from build123d import *

# Parameters (mm, degrees)
BOSS_EXTRUDE1_DEPTH                             = 38.1
BOSS_EXTRUDE2_START                             = -3.175
BOSS_EXTRUDE2_DEPTH                             = 3.175
CBORE_FOR_2_PAN_HEAD_MACHINE_SCREW1_D           = 2.7051
CBORE_FOR_2_PAN_HEAD_MACHINE_SCREW1_DEPTH       = 2.667
CBORE_FOR_2_PAN_HEAD_MACHINE_SCREW1_CBORE_D     = 4.7625
CBORE_FOR_2_PAN_HEAD_MACHINE_SCREW1_CBORE_DEPTH = 1.5748
CBORE_START                                     = 26.4287
CBORE_FOR_2_PAN_HEAD_MACHINE_SCREW2_OUT_R       = 2.38125
CBORE_FOR_2_PAN_HEAD_MACHINE_SCREW2_DEPTH       = 1.574800075
CBORE_START_2                                   = 25.300372244
CBORE_FOR_2_PAN_HEAD_MACHINE_SCREW2_2_O_R       = 1.35255
CBORE_FOR_2_PAN_HEAD_MACHINE_SCREW2_2_DEPTH     = 1.128327756
CBORE_START_3                                   = -28.003500101
CBORE_FOR_2_PAN_HEAD_MACHINE_SCREW3_OUT_R       = 2.38125
CBORE_FOR_2_PAN_HEAD_MACHINE_SCREW3_DEPTH       = 1.574800101
CBORE_START_4                                   = -26.4287
CBORE_FOR_2_PAN_HEAD_MACHINE_SCREW3_2_O_R       = 1.35255
CBORE_FOR_2_PAN_HEAD_MACHINE_SCREW3_2_DEPTH     = 1.128327733
CUT_EXTRUDE1_REACH                              = 56.955
SKETCH20_R                                      = 7.27
HOLE1_AT_2_COUNT                                = 2
HOLE1_AT_2_PITCH                                = 19
F_0_CLEARANCE_HOLE1_D                           = 1.8542
CHAMFER1_SIZE                                   = 1.27


# Read off the part's stored shape, not the designer's step: CBORE for #2 Pan Head Machine Screw2, CBORE for #2 Pan Head Machine Screw3
with BuildPart() as part:
    # Sketch1 → Boss-Extrude1 (new body)
    with BuildSketch(Plane.XY):
        with BuildLine():
            Line((15.182514888, 23.53056), (-15.182514888, 23.53056))
            ThreePointArc((-15.182514888, 23.53056), (0, -28.0035), (15.182514888, 23.53056))
        make_face()
        with BuildLine():
            Line((14.375329435, 20.86356), (-14.375329435, 20.86356))
            ThreePointArc((-14.375329435, 20.86356), (0, -25.3365), (14.375329435, 20.86356))
        make_face(mode=Mode.SUBTRACT)
    extrude(amount=BOSS_EXTRUDE1_DEPTH)

    # Sketch10 → Boss-Extrude2 (add)
    with BuildSketch(Plane.XY.offset(38.1).offset(BOSS_EXTRUDE2_START)):
        with BuildLine():
            Line((15.182514888, 23.53056), (-15.182514888, 23.53056))
            ThreePointArc((-15.182514888, 23.53056), (0, -28.0035), (15.182514888, 23.53056))
        make_face()
    extrude(amount=BOSS_EXTRUDE2_DEPTH)

    # CBORE for #2 Pan Head Machine Screw1
    with Locations(Plane(origin=(-7.747359339, 23.53056, 10.2108), x_dir=(0, 0, -1), z_dir=(0, 1, 0))):
        with Locations((1.8613, -7.747359339)):
            CounterBoreHole(CBORE_FOR_2_PAN_HEAD_MACHINE_SCREW1_D / 2, CBORE_FOR_2_PAN_HEAD_MACHINE_SCREW1_CBORE_D / 2, CBORE_FOR_2_PAN_HEAD_MACHINE_SCREW1_CBORE_DEPTH, depth=CBORE_FOR_2_PAN_HEAD_MACHINE_SCREW1_DEPTH)

    # CBORE for #2 Pan Head Machine Screw2 out → CBORE for #2 Pan Head Machine Screw2 (cut)
    with BuildSketch(Plane(origin=(0, 0, 0), x_dir=(0.8660254037844416, 0.4999999999999948, 0), z_dir=(0.4999999999999948, -0.8660254037844417, 0)).offset(CBORE_START)):
        with Locations((0, 10.2108)):
            Circle(CBORE_FOR_2_PAN_HEAD_MACHINE_SCREW2_OUT_R)
    extrude(amount=CBORE_FOR_2_PAN_HEAD_MACHINE_SCREW2_DEPTH, mode=Mode.SUBTRACT)

    # CBORE for _2 Pan Head Machine Screw2 2 o → CBORE for _2 Pan Head Machine Screw2 2 (cut)
    with BuildSketch(Plane(origin=(0, 0, 0), x_dir=(0.8660254037844416, 0.4999999999999948, 0), z_dir=(0.4999999999999948, -0.8660254037844417, 0)).offset(CBORE_START_2)):
        with Locations((0, 10.2108)):
            Circle(CBORE_FOR_2_PAN_HEAD_MACHINE_SCREW2_2_O_R)
    extrude(amount=CBORE_FOR_2_PAN_HEAD_MACHINE_SCREW2_2_DEPTH, mode=Mode.SUBTRACT)

    # CBORE for #2 Pan Head Machine Screw3 out → CBORE for #2 Pan Head Machine Screw3 (cut)
    with BuildSketch(Plane.YZ.offset(CBORE_START_3)):
        with Locations((0, 10.2108)):
            Circle(CBORE_FOR_2_PAN_HEAD_MACHINE_SCREW3_OUT_R)
    extrude(amount=CBORE_FOR_2_PAN_HEAD_MACHINE_SCREW3_DEPTH, mode=Mode.SUBTRACT)

    # CBORE for _2 Pan Head Machine Screw3 2 o → CBORE for _2 Pan Head Machine Screw3 2 (cut)
    with BuildSketch(Plane.YZ.offset(CBORE_START_4)):
        with Locations((0, 10.2108)):
            Circle(CBORE_FOR_2_PAN_HEAD_MACHINE_SCREW3_2_O_R)
    extrude(amount=CBORE_FOR_2_PAN_HEAD_MACHINE_SCREW3_2_DEPTH, mode=Mode.SUBTRACT)

    # Sketch20 → Cut-Extrude1 (cut, up to next)
    with BuildSketch(Plane.XY.offset(38.1), mode=Mode.PRIVATE) as cut_extrude1_sk1:
        Circle(SKETCH20_R)
    cut_extrude1_tool1 = extrude(cut_extrude1_sk1.sketch, amount=-CUT_EXTRUDE1_REACH, mode=Mode.PRIVATE) & part.part
    add(cut_extrude1_tool1.solids().sort_by_distance((0, 0, 38.1))[0], mode=Mode.SUBTRACT)

    # Sketch22 → Hole1 (revolve, cut)
    with BuildSketch(Plane(origin=(9.5, 0, 34.925), x_dir=(0, 1, 0), z_dir=(1, 0, 0))):
        Polygon((0, 0), (0, 2.921), (1.4986, 2.921), (1.6383, 0), align=None)
    hole1 = revolve(axis=Axis((9.5, 0, 144.925), (0, 0, -1)), mode=Mode.SUBTRACT)

    # Hole1 at 2: Hole1 ×2
    with Locations(*[(-i * HOLE1_AT_2_PITCH, 0, 0) for i in range(1, HOLE1_AT_2_COUNT)]):
        add(hole1, mode=Mode.SUBTRACT)

    # #0 Clearance Hole1 (through all)
    with Locations(Plane(origin=(0, 0, 34.925), x_dir=(-1, 0, 0), z_dir=(0, 0, -1))):
        with Locations((-9.5, 0), (9.5, 0)):
            Hole(F_0_CLEARANCE_HOLE1_D / 2)

    # Chamfer1
    chamfer1_edges = [part.edges().sort_by_distance(p)[0] for p in [
        (0, -25.3365, 0),
        (0, 20.86356, 0),
    ]]
    chamfer(chamfer1_edges, length=CHAMFER1_SIZE)


solid = part.part
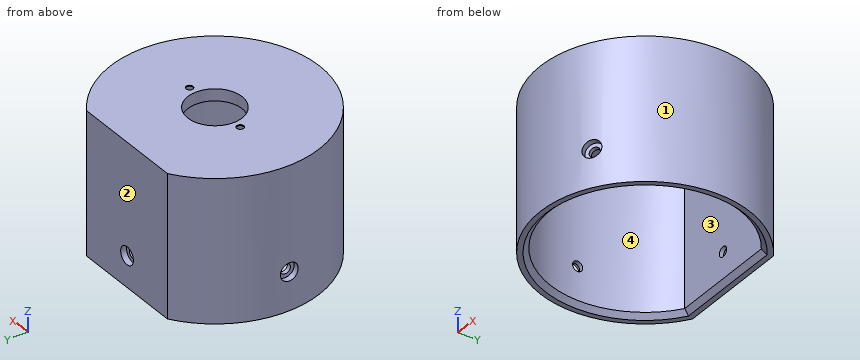
Geometry: final body of the model. Coordinates: model frame, mm. Face numbers are marked on the shaded views. Coordinates: 2 decimals unless noted, no trailing zeros. Order: outer loops, then holes, each group sorted by start corner. A loop starts at its lowest first (then second) coordinate and runs counter-clockwise, first axis right, second up. Notation, with made-up numbers: M 35,11.25 L 63,11.25 A14 cw 63,27.25 Z; hole C 46,-28.5 d8. An arc over 180 degrees is marked long. One line per question, with ' | ' between items. Start each with the question number.
Item 1: Pin query (flat end, axial travel): pin 1 Ø1.7 at (x, y) = (9.5, 0) entering from -Z; pin 2 Ø12 at (y, z) = (-21, 12) entering from +X; pin 3 Ø2 at (y, z) = (-6.5, 21) entering from +X; pin 4 Ø5 at (y, z) = (-22.5, 28.5) entering from -X. Return the tip coordinate at first contact, or that it passes through.
Item 2: Cut plane B-B, the plane y = 0. Count the separate pieces of the cut face and the enclosed holes in it, then the cut area to 3 significant figures.
Item 3: Draft query along X for the marked faces 1, 2, 3 and 4. Return one class per face: released by +X, released by -X, zero draft, split by the parting line, or undercut.
Item 4: Cut plane A-A, the plane z = 16.5. Return the cut outline in (x, y).
Item 5: Ray query, probe 1 along X at (y, z) = (0, 23); probe 2 along X at (y, z) = (0, 8.5); probe 3 along Z at (x, y) = (-27.35, 0). Return the intervals inside material, ascending. Write a range as [from, to].
A:
1) pin 1: passes through | pin 2: stops at x = 23.65 | pin 3: stops at x = 27.46 | pin 4: stops at x = -19.6
2) separate pieces: 5 | enclosed holes: 0 | area: 287 mm2
3) face 1: split by the parting line | face 2: zero draft | face 3: undercut | face 4: undercut
4) outline: M -15.18,23.53 A28 ccw long 15.18,23.53 Z; hole M -14.38,20.86 A25.34 ccw long 14.38,20.86 Z
5) probe 1: x = [-28, -25.34], [25.34, 28] | probe 2: x = [-26.43, -25.34], [25.34, 28] | probe 3: z = [0, 7.83], [12.59, 38.1]
